Autodesk Inventor part; units mm, degrees
ref_plane "YZ Plane" through (0, 0, 0) normal (1, 0, 0) x (0, 1, 0)
ref_plane "XZ Plane" through (0, 0, 0) normal (0, 1, 0) x (-1, 0, 0)
ref_plane "XY Plane" through (0, 0, 0) normal (0, 0, 1) x (1, 0, 0)
sketch "스케치1" plane through (0, 0, 0) normal (0, 0, 1) x (1, 0, 0)
  circle A0 centre (0, 0) radius 27
  line L0 (-22.5, -22.5) -> (22.5, -22.5)
  line L1 (22.5, -22.5) -> (22.5, 22.5)
  line L2 (22.5, 22.5) -> (-22.5, 22.5)
  line L3 (-22.5, 22.5) -> (-22.5, -22.5)
  line L4 (-22.5, -22.5) -> (22.5, 22.5) construction
  line L5 (22.5, -22.5) -> (-22.5, 22.5) construction
  point P0 (-22.5, 14.9248)
  point P1 (-22.5, -14.9248)
  point P2 (-14.9248, -22.5)
  point P3 (14.9248, -22.5)
  point P4 (22.5, -14.9248)
  point P5 (22.5, 14.9248)
  point P6 (14.9248, 22.5)
  point P7 (-14.9248, 22.5)
  dimension "d0" = 54
  dimension "d5" = 45
  dimension "d6" = 45
extrude "돌출1" add sketch "스케치1" along normal blind 15 contours L1 A0 L0 L3 L2
sketch "스케치2" plane through (0, 0, 15) normal (0, 0, 1) x (1, 0, 0)
  point P0 (0, 0)
sketch "스케치3" plane through (0, 0, 15) normal (0, 0, 1) x (1, 0, 0)
  circle A0 centre (0, 0) radius 3.9
  line L0 (-2.492, 3) -> (2.492, 3)
  dimension "d7" = 7.8
  dimension "d8" = 3
extrude "돌출2" add sketch "스케치3" along normal blind 20 contours A0 L0 picked at (1.186, -0.6989)
extrude "돌출3" add sketch "스케치3" along normal blind 5 contours L0 A0 picked at (-0.5796, 3.1636)
fillet "모깎기1" radius 2 1 edges at (-2.492, -3, 15)
properties part number "손잡이 축"
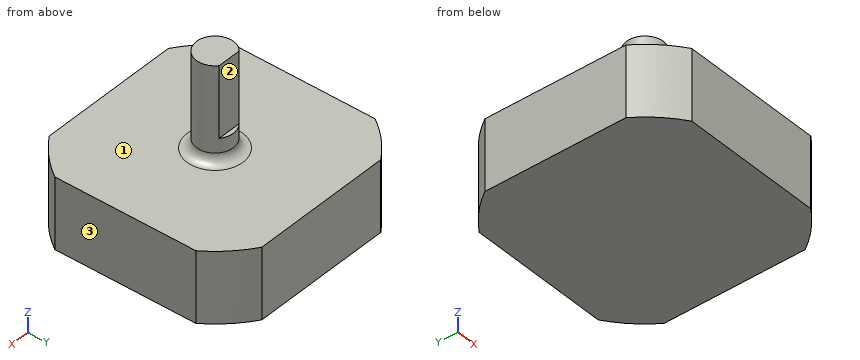
Part model, mm, in its own coordinate system. Face numbers are marked on the shaded views. A direction names the side the tool comes from. Coordinates: 2 decimals unless noted, no trailing zeros. Order: outer loops, then holes, each group sorted by start corner. A loop starts at its lowest first (then second) coordinate and runs counter-clockwise, first axis right, second up.
(1) Slice it at D-D, the plane y = -8.5. Write the cut outline in (x, z), and give its area (3 significant figures).
Check sheet entries:
outline: (-22.5, 0) - (22.5, 0) - (22.5, 15) - (-22.5, 15) - close
area: 675 mm2
(2) Slice it at A-A, the plane y = 0. Write the cut outline in (x, z), and give its area (3 significant figures).
Check sheet entries:
outline: (-22.5, 0) - (22.5, 0) - (22.5, 15) - (5.9, 15) arc R2 cw to (3.9, 17) - (3.9, 35) - (-3.9, 35) - (-3.9, 17) arc R2 cw to (-5.9, 15) - (-22.5, 15) - close
area: 833 mm2
(3) Pin check, flat tips, straight feed: pin 1 Ø10 at (y, z) = (-10, 26) entering from +X; pin 2 Ø4 at (x, z) = (-1, 27) entering from +Y. Stop position of each tip, or through.
Check sheet entries:
pin 1: passes through
pin 2: stops at y = 3
(4) Slice it at C-C, the plane z = 9. Write the cut outline in (x, y).
Check sheet entries:
outline: (-22.5, -14.92) arc R27 ccw to (-14.92, -22.5) - (14.92, -22.5) arc R27 ccw to (22.5, -14.92) - (22.5, 14.92) arc R27 ccw to (14.92, 22.5) - (-14.92, 22.5) arc R27 ccw to (-22.5, 14.92) - close
(5) Tool access for the marked faces 1, 2 and 3: list every direction of +Z, -Z, +X, -X, +Y, -Y with a clear straight run to the whole face (end or side of a thin tool).
Check sheet entries:
face 1: +Z
face 2: +Z, +X, -X, +Y
face 3: +Z, -Z, +X, +Y, -Y
(6) Slice it at B-B, the plane x = 0. Write the cut outline in (y, z).
Check sheet entries:
outline: (-22.5, 0) - (22.5, 0) - (22.5, 15) - (5.9, 15) arc R2 cw to (3.9, 17) - (3.9, 20) - (3, 20) - (3, 35) - (-3.9, 35) - (-3.9, 17) arc R2 cw to (-5.9, 15) - (-22.5, 15) - close
(7) Probe L1, parallel to Z at x = 11, y = -0.5; L2, parallel to X at y = -17, z = 9.5; L3, parallel to X at y = -19.5, z = 3. List the from-to ranges inside material, lowest first.
Check sheet entries:
L1: z = 0 to 15
L2: x = -20.98 to 20.98
L3: x = -18.67 to 18.67
